Work out the finished part from the listing and answer in its coordinate system (mm). Face numbers are marked on the shaded views. A direction names the side the tool comes from. Coordinates: 2 decimals unless noted, no trailing zeros. Write each loop counter-clockwise with the first axis right and the second up, starting at its lowest first coordinate (ties: lowest second). Pieces come first, ordered by that corner, then holes. Notation, with made-up numbers: M 33.25,48 L 42.25,48 A16 ccw 42.25,79 Z; hole C 46.5,-19 d6. An arc over 180 degrees is marked long. Answer as CSV lines item,"result". Start each with the question number.
(1) A cutting plane is placed at A-A on y = -7.25. Give the vertices of the cut face in (x, z).
(2) Find the intervals of material crossed by L1, parallel to Z at x = -8, y = -4.25; L2, parallel to Y at x = 17, z = 5.75; L3, parallel to X at y = -4.75, z = -1, in increasing order. Write a range as [from, to].
(3) A cutting plane is placed at C-C on z = -7.25. Give the vertices of the cut face in (x, y).
(4) Flat-ended cylindrical pins translate along their axes: P1, Ø10, axis at x = 40, z = 2.5, coming from the +Y side; P2, Ø3, axis at y = -17, z = -8.5, coming from the -X side; P3, Ø12, axis at x = 42, y = -18.5, coming from the -Z side; P4, Ø3, axis at y = -5, z = 6, coming from the +X side. Find the tip coordinate at first contact, or state that the pin passes through.
(5) A cutting plane is placed at B-B on x = -3.5. Give the vertices of the cut face in (y, z), then the cut area to 3 significant figures.
(6) The mould has two halves that part along Z. Classify the marked faces 3, 4 and 5: released by +Z, released by -Z, zero draft, split by the parting line, or undercut.
(7) For the marked faces 1 and 2, determine the directions among +Z, -Z, +X, -X, +Y, -Y from which every point of the face is accessible in a straight line to the end or side of a thin tool.
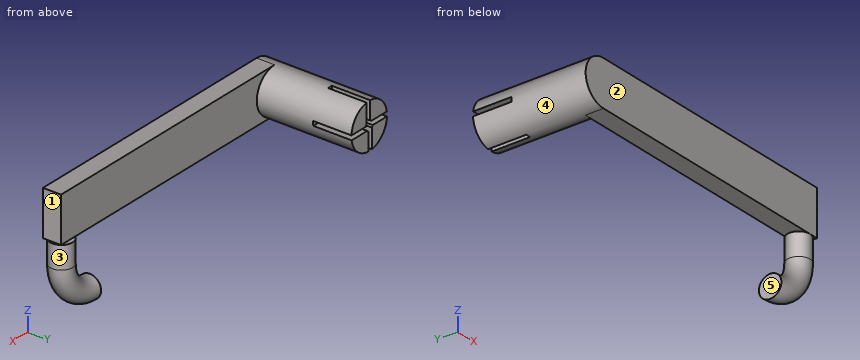
from build123d import *

# Parameters (mm, degrees)
SKETCH083_R     = 5
PAD031_DEPTH    = 25
SKETCH084_W     = 60
SKETCH084_H     = 10
PAD032_DEPTH    = 4
SKETCH085_R     = 2.5
POCKET027_DEPTH = 8.5
SKETCH088_R     = 1
POCKET028_DEPTH = 8.5


with BuildPart() as part:
    # Sketch083 → Pad031 (new body)
    with BuildSketch(Plane.XZ):
        Circle(SKETCH083_R)
    extrude(amount=PAD031_DEPTH)

    # Sketch084 (on Face3 of Pad031) → Pad032 (join)
    with BuildSketch(Plane.XZ.offset(25)):
        with Locations((30, 0)):
            Rectangle(SKETCH084_W, SKETCH084_H)
    extrude(amount=-PAD032_DEPTH)

    # AdditivePipe: sweep along a path in Sketch086
    with BuildLine(Plane.XZ.offset(23)) as additivepipe_path:
        ThreePointArc((50, -18), (55.656854, -15.656854), (58, -10))
        Line((58, -10), (58, -5))
    # Sketch085 (on Face4 of Pad032) → AdditivePipe (sweep)
    with BuildSketch(Plane(origin=(0, 0, -5), x_dir=(1, 0, 0), z_dir=(0, 0, -1))):
        with Locations((58, 22.5)):
            Circle(SKETCH085_R)
    sweep(path=additivepipe_path.line)

    # Sketch087 (on Face2 of AdditivePipe) → Pocket027 (cut)
    with BuildSketch(Plane(origin=(0, 0, 0), x_dir=(1, 0, 0), z_dir=(0, 1, 0))):
        Polygon((-0.75, 6.25), (-0.75, 0.25), (-6.25, 0.25), (-6.25, -0.75), (-0.25, -0.75), (-0.25, -6.25), (0.75, -6.25), (0.75, -0.25), (6.25, -0.25), (6.25, 0.75), (0.25, 0.75), (0.25, 6.25), align=None)
    extrude(amount=-POCKET027_DEPTH, mode=Mode.SUBTRACT)

    # Sketch088 → Pocket028 (cut)
    with BuildSketch(Plane(origin=(0, 0, 0), x_dir=(-1, 0, 0), z_dir=(0, 1, 0))):
        Circle(SKETCH088_R)
    extrude(amount=-POCKET028_DEPTH, mode=Mode.SUBTRACT)


with BuildPart() as part_1:
    # Body013 placement: moved
    add(part.part.moved(Location((-12, 0, 2))))


solid = part_1.part
Here are the results:
1,outline,"M -16.99,1.75 A5 ccw -12.75,-2.94 L -12.75,1.34 A1 cw -12.97,1.75 Z; M -16.94,2.75 L -12.66,2.75 A1 cw -12.25,2.97 L -12.25,6.99 A5 ccw Z; M -11.75,-2.99 A5 ccw -7.06,1.25 L -11.34,1.25 A1 cw -11.75,1.03 Z; M -11.25,2.66 A1 cw -11.03,2.25 L -7.01,2.25 A5 ccw -11.25,6.94 Z"
2,L1,"z = [-1, 1.25], [2.25, 5]"
2,L2,"y = [-25, -21]"
2,L3,"x = [-16, -12.75], [-11.75, -8]"
3,outline,"C 46,-22.5 d5"
4,P1,"stops at y = -21"
4,P2,"passes through"
4,P3,"stops at z = -18.5"
4,P4,"stops at x = -7.67"
5,outline,"M -25,-3 L -21,-3 L -21,7 L -25,7 Z"
5,area,"40.0 mm^2"
6,face 3,"undercut"
6,face 4,"split by the parting line"
6,face 5,"zero draft"
7,face 1,"+Z, +X, +Y, -Y"
7,face 2,"+Z, -Z, +X, -X, -Y"
